Geometry: see drawing. Coordinates: mm, zero at the bounding-box minimum. A direction names the side the tool comes from. Round coordinates to 2 decimals unless told otherwise and drop trailing zeros. Order: outer loops, then holes, each group sorted by start corner. A loop starts at its lowest first (then second) coordinate and runs counter-clockwise, first axis right, second up. Notation, with made-up numbers: (-8, 0.5) -> (39, 0.5) arc R29 cw to (39, 28.5) -> close; hole circle Ø7 at (50, 12). An arc over 180 degrees is marked (long way). One line per item, written item: value. Start each with the question number.
1) Mould query, pull axis Y, two halves, no side actions, for the marked faces 1, 2, 3 and 4. Classes: pulls with the +Y half, pulls with the -Y half, needs draft (parallel to the pull), parting line crosses it, or undercut.
2) Section B-B (y = 33.5). Return the cut outline in (x, z).
3) Reachability of the marked faces 5, 6 and 7 from +Z, -Z, +X, -X, +Y, -Y: full face, straight path, thin tool, end or side. Return the list, or none.
4) Pin query (flat end, axial travel): P1, Ø6, axis at y = 48, z = 15.5, coming from the +X side; P2, Ø8.5, axis at y = 53, z = 13, coming from the -X side; P3, Ø3, axis at y = 28, z = 11.5, coming from the +X side. Return the tip coordinate at first contact, or that it passes through.
5) Section D-D (x = 54). Return the cut outline in (y, z).
6) Ray query, L1, parallel to Y at x = 3, z = 1.05; L2, parallel to X at y = 64, z = 0.5; L3, parallel to Y at x = 49.5, z = 13.75. Return the intervals inside material, ascending.
7) Section A-A (z = 4). Return the cut outline in (x, y).
8) Section C-C (z = 17). Return the cut outline in (x, y), and give its area (3 significant figures).
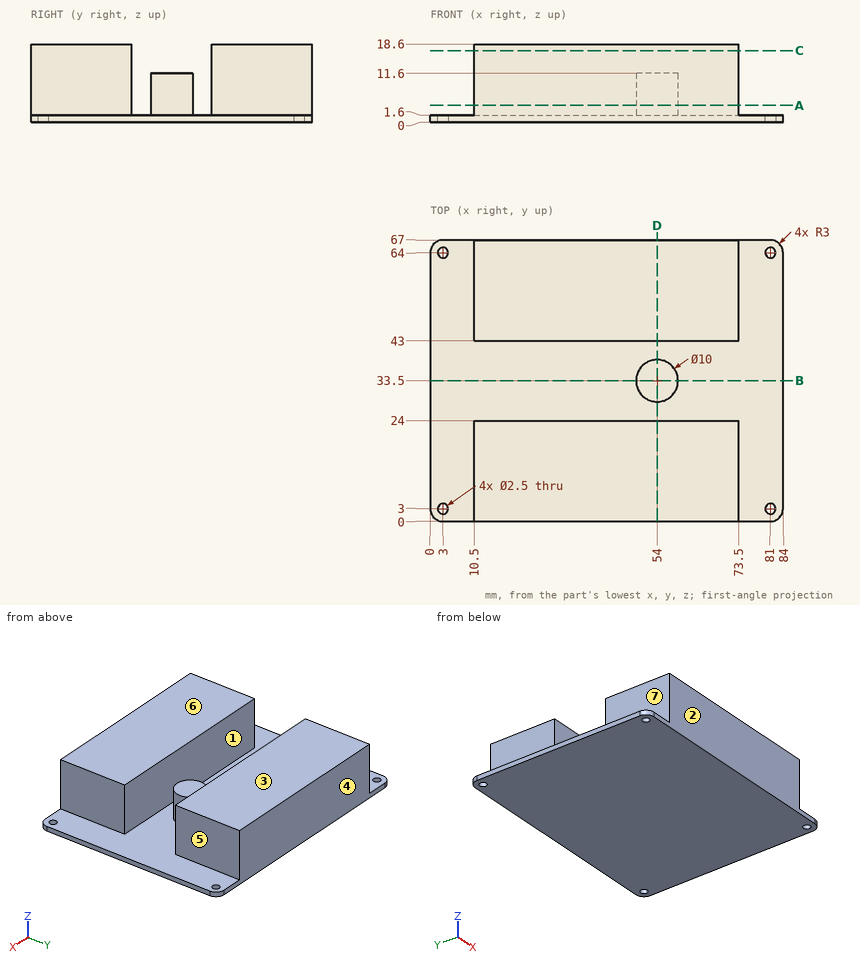
Findings:
1. face 1: undercut
1. face 2: pulls with the -Y half
1. face 3: needs draft
1. face 4: pulls with the +Y half
2. outline: (0, 0) -> (84, 0) -> (84, 1.6) -> (59, 1.6) -> (59, 11.6) -> (49, 11.6) -> (49, 1.6) -> (0, 1.6) -> close
3. face 5: +Z, +X, +Y, -Y
3. face 6: +Z, +X, -X, +Y, -Y
3. face 7: +Z, -X, +Y, -Y
4. P1: x = 73.5
4. P2: x = 10.5
4. P3: x = 57
5. outline: (0, 0) -> (67, 0) -> (67, 18.6) -> (43, 18.6) -> (43, 1.6) -> (38.5, 1.6) -> (38.5, 11.6) -> (28.5, 11.6) -> (28.5, 1.6) -> (24, 1.6) -> (24, 18.6) -> (0, 18.6) -> close
6. L1: 0 to 1.75, 4.25 to 62.75, 65.25 to 67
6. L2: 0 to 1.75, 4.25 to 79.75, 82.25 to 84
6. L3: 0 to 24, 43 to 67
7. outline: (10.5, 0) -> (73.5, 0) -> (73.5, 24) -> (10.5, 24) -> close; (10.5, 43) -> (73.5, 43) -> (73.5, 67) -> (10.5, 67) -> close; circle Ø10 at (54, 33.5)
8. outline: (10.5, 0) -> (73.5, 0) -> (73.5, 24) -> (10.5, 24) -> close; (10.5, 43) -> (73.5, 43) -> (73.5, 67) -> (10.5, 67) -> close
8. area: 3,020 mm2
